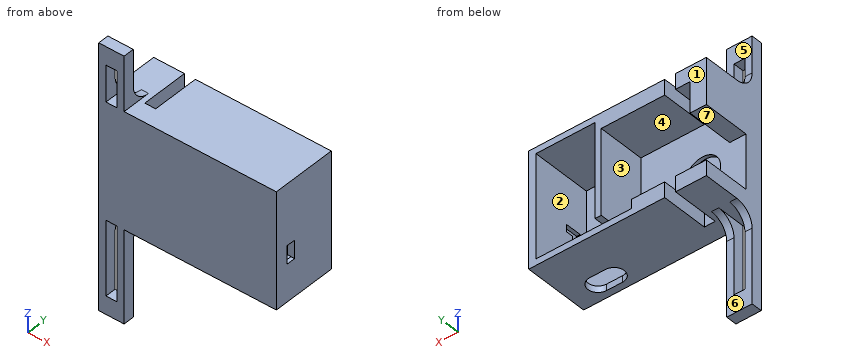
```python
from build123d import *

# Parameters (mm, degrees)
SKETCH_1_W           = 49
SKETCH_1_H           = 32
EXTRUDE_2_DEPTH      = 18
SKETCH_6_W           = 24.5
SKETCH_6_H           = 23.5
CUT_EXTRUDE_1_DEPTH  = 13
SKETCH_7_W           = 16.3
SKETCH_7_H           = 28.5
CUT_EXTRUDE_2_DEPTH  = 16.5
SKETCH_8_W           = 3
SKETCH_8_H           = 32
CUT_EXTRUDE_3_DEPTH  = 13
SKETCH_12_W          = 15
SKETCH_12_H          = 13
CUT_EXTRUDE_5_DEPTH  = 58.690987164
SKETCH_13_W          = 10
SKETCH_13_H          = 2.5
CUT_EXTRUDE_6_DEPTH  = 13
CUT_EXTRUDE_7_DEPTH  = 61.332930477
SKETCH_15_W          = 7
SKETCH_15_H          = 25.5
EXTRUDE_3_DEPTH      = 3
SKETCH_16_W          = 7
SKETCH_16_H          = 15
EXTRUDE_4_DEPTH      = 3
FILLET_1_R           = 5
SKETCH_17_W          = 3
SKETCH_17_H          = 10
SKETCH_17_H_2        = 20.5
CUT_EXTRUDE_8_DEPTH  = 78.661122835
SKETCH_19_R          = 5
CUT_EXTRUDE_9_DEPTH  = 1
CUT_EXTRUDE_10_DEPTH = 1
SKETCH_25_W          = 5
SKETCH_25_H          = 2.5
CUT_EXTRUDE_13_DEPTH = 78.034083366


with BuildPart() as part:
    # 草图1 → 凸台-拉伸2 (new body)
    with BuildSketch(Plane(origin=(0, 0, 0), x_dir=(1, 0, 0), z_dir=(0, 1, 0))):
        with Locations((24.5, 16)):
            Rectangle(SKETCH_1_W, SKETCH_1_H)
    extrude(amount=EXTRUDE_2_DEPTH)

    # 草图6 → 切除-拉伸1 (cut)
    with BuildSketch(Plane(origin=(0, 18, 0), x_dir=(1, 0, 0), z_dir=(0, 1, 0))):
        with Locations((16.75, 16)):
            Rectangle(SKETCH_6_W, SKETCH_6_H)
    extrude(amount=-CUT_EXTRUDE_1_DEPTH, mode=Mode.SUBTRACT)

    # 草图7 → 切除-拉伸2 (cut)
    with BuildSketch(Plane(origin=(0, 18, 0), x_dir=(1, 0, 0), z_dir=(0, 1, 0))):
        with Locations((38.85, 16)):
            Rectangle(SKETCH_7_W, SKETCH_7_H)
    extrude(amount=-CUT_EXTRUDE_2_DEPTH, mode=Mode.SUBTRACT)

    # 草图8 → 切除-拉伸3 (cut)
    with BuildSketch(Plane(origin=(0, 18, 0), x_dir=(1, 0, 0), z_dir=(0, 1, 0))):
        with Locations((10, 16)):
            Rectangle(SKETCH_8_W, SKETCH_8_H)
    extrude(amount=-CUT_EXTRUDE_3_DEPTH, mode=Mode.SUBTRACT)

    # 草图12 → 切除-拉伸5 (cut, through all)
    with BuildSketch(Plane(origin=(4.5, 0, 0), x_dir=(0, 0, -1), z_dir=(1, 0, 0))):
        with Locations((20.25, 11.5)):
            Rectangle(SKETCH_12_W, SKETCH_12_H)
    extrude(amount=-CUT_EXTRUDE_5_DEPTH, mode=Mode.SUBTRACT)

    # 草图13 → 切除-拉伸6 (cut)
    with BuildSketch(Plane(origin=(0, 18, 0), x_dir=(1, 0, 0), z_dir=(0, 1, 0))):
        with Locations((25.7, 29)):
            Rectangle(SKETCH_13_W, SKETCH_13_H)
    extrude(amount=-CUT_EXTRUDE_6_DEPTH, mode=Mode.SUBTRACT)

    # 草图14 → 切除-拉伸7 (cut, through all)
    with BuildSketch(Plane(origin=(0, 0, -1.75), x_dir=(-1, 0, 0), z_dir=(0, 0, -1))):
        with BuildLine():
            Line((-41.05, 7.5), (-36.65, 7.5))
            ThreePointArc((-36.65, 7.5), (-33.85, 4.7), (-36.65, 1.9))
            Line((-36.65, 1.9), (-41.05, 1.9))
            ThreePointArc((-41.05, 1.9), (-43.85, 4.7), (-41.05, 7.5))
        make_face()
    extrude(amount=CUT_EXTRUDE_7_DEPTH, mode=Mode.SUBTRACT)

    # 草图15 → 凸台-拉伸3 (add)
    with BuildSketch(Plane(origin=(0, 0, 0), x_dir=(-1, 0, 0), z_dir=(0, -1, 0))):
        with Locations((-3.5, 44.75)):
            Rectangle(SKETCH_15_W, SKETCH_15_H)
    extrude(amount=-EXTRUDE_3_DEPTH)

    # 草图16 → 凸台-拉伸4 (add)
    with BuildSketch(Plane.XZ):
        with Locations((3.5, 7.5)):
            Rectangle(SKETCH_16_W, SKETCH_16_H)
    extrude(amount=-EXTRUDE_4_DEPTH)

    # 圆角1
    fillet_1_edges = [part.edges().sort_by_distance(p)[0] for p in [
        (3.5, 3, -32),
        (3.5, 3, 0),
    ]]
    fillet(fillet_1_edges, radius=FILLET_1_R)

    # 草图17 → 切除-拉伸8 (cut, through all)
    with BuildSketch(Plane(origin=(0, 0, 0), x_dir=(-1, 0, 0), z_dir=(0, -1, 0))):
        with Locations((-3.5, -5)):
            Rectangle(SKETCH_17_W, SKETCH_17_H)
        with Locations((-3.5, 42.25)):
            Rectangle(SKETCH_17_W, SKETCH_17_H_2)
    extrude(amount=-CUT_EXTRUDE_8_DEPTH, mode=Mode.SUBTRACT)

    # 草图19 → 切除-拉伸9 (cut)
    with BuildSketch(Plane(origin=(0, 5, 0), x_dir=(1, 0, 0), z_dir=(0, 1, 0))):
        with Locations(Location((12, 17.75, 0), (0, 0, 270))):
            Circle(SKETCH_19_R)
    extrude(amount=-CUT_EXTRUDE_9_DEPTH, mode=Mode.SUBTRACT)

    # 草图20 → 切除-拉伸10 (cut)
    with BuildSketch(Plane.ZY.offset(-47)):
        Polygon((-23.75, 3.5), (-14.75, 3.5), (-14.75, 6), (-14.75, 8), (-16.75, 8), (-16.75, 6), (-21.75, 6), (-21.75, 8), (-23.75, 8), (-23.75, 6), align=None)
    extrude(amount=-CUT_EXTRUDE_10_DEPTH, mode=Mode.SUBTRACT)

    # 草图25 → 切除-拉伸13 (cut, through all)
    with BuildSketch(Plane.ZY.offset(-48)):
        with Locations((-19.25, 4.75)):
            Rectangle(SKETCH_25_W, SKETCH_25_H)
    extrude(amount=-CUT_EXTRUDE_13_DEPTH, mode=Mode.SUBTRACT)


solid = part.part
```
Geometry check sheet. Reference: the model listing, model coordinates, mm. Face numbers are marked on the shaded views. A direction names the side the tool comes from. Give positions to 0.01 mm unless a question says otherwise; leave off trailing zeros. Write each loop counter-clockwise with the first axis right and the second up, starting at its lowest first coordinate (ties: lowest second). Pieces come first, ordered by that corner, then holes. Notation, with made-up numbers: (54, 41.25) -> (79, 41.25) arc R12 cw to (79, 59.25) -> close; hole circle Ø4 at (24, -17). An arc over 180 degrees is marked (long way). Use one line per item in the form item = value.
Item 1: Sectioned sample at C-C on x = 6. Enter the section's corners in (y, z).
Results list:
outline = (0, -57.5) -> (3, -57.5) -> (3, -37) arc R5 cw to (8, -32) -> (18, -32) -> (18, -27.75) -> (5, -27.75) -> (5, -4.25) -> (18, -4.25) -> (18, 0) -> (8, 0) arc R5 cw to (3, 5) -> (3, 15) -> (0, 15) -> close
Item 2: Sectioned sample at D-D on z = -31. Enter the section's corners in (x, y), plus the area to 3 significant figures.
Results list:
outline = (0, 0) -> (49, 0) -> (49, 18) -> (11.5, 18) -> (11.5, 5) -> (8.5, 5) -> (8.5, 18) -> (0, 18) -> close; hole (36.65, 1.9) -> (41.05, 1.9) arc R2.8 ccw to (41.05, 7.5) -> (36.65, 7.5) arc R2.8 ccw to start
area = 794 mm2
Item 3: Sectioned sample at A-A on z = -17.75. Enter the section's corners in (x, y).
Results list:
outline = (0, 0) -> (49, 0) -> (49, 3.5) -> (47, 3.5) -> (47, 1.5) -> (30.7, 1.5) -> (30.7, 18) -> (29, 18) -> (29, 5) -> (17, 5) -> (17, 4) -> (7, 4) -> (7, 5) -> (0, 5) -> close; (47, 6) -> (49, 6) -> (49, 18) -> (47, 18) -> close
Item 4: Sectioned sample at B-B on y = 12.5. Enter the section's corners in (x, z), plus the area to 3 significant figures.
Results list:
outline = (0, -32) -> (8.5, -32) -> (8.5, -27.75) -> (0, -27.75) -> close; (0, -12.75) -> (4.5, -12.75) -> (4.5, -4.25) -> (8.5, -4.25) -> (8.5, 0) -> (0, 0) -> close; (11.5, -32) -> (49, -32) -> (49, 0) -> (11.5, 0) -> (11.5, -4.25) -> (29, -4.25) -> (29, -27.75) -> (30.7, -27.75) -> (30.7, -1.75) -> (47, -1.75) -> (47, -30.25) -> (20.7, -30.25) -> (20.7, -27.75) -> (11.5, -27.75) -> close
area = 410 mm2
Item 5: Access from +Z, -Z, +X, -X, +Y, -Y to the whole of each face (thin tool, end or side, straight path). Record for the marked faces 4, 5, 6 and 7.
Results list:
face_4 = +Y
face_5 = +Z, +X, -X, +Y
face_6 = -Z, +X, -X, +Y
face_7 = -X, +Y
Item 6: Scan lines: line 1 (X direction, y = 10.75, z = -8.5); line 2 (Z direction, x = 3.5, y = 13.5); line 3 (X direction, y = 4.65, z = -17.75). Record each from-to range of solid material in increasing order.
Results list:
line_1 = 0 to 4.5, 29 to 30.7, 47 to 49
line_2 = -32 to -27.75, -12.75 to 0
line_3 = 0 to 7, 17 to 30.7
Item 7: Depth check by flat-ended pin: pin 1 Ø2 at (x, y) = (32.5, 8) entering from +Z; pin 2 Ø11.5 at (x, z) = (12, -17.75) entering from +Y; pin 3 Ø9 at (y, z) = (5, -37) entering from +X. Enter the tip coordinate at first touch or a pass-through.
Results list:
pin_1 = 0
pin_2 = 5
pin_3 = 7
Item 8: Mould release check, pull along Z, two halves, no side actions. Record for the marked faces 1, 2 and 3: released by +Z, released by -Z, zero draft, split by the parting line, or undercut.
Results list:
face_1 = zero draft
face_2 = undercut
face_3 = undercut
